Work out the finished part from the listing and answer in its coordinate system (mm). Round coordinates to 2 decimals unless told otherwise and drop trailing zeros. Answer as CSV lines item,"result". Start each with the question number.
Q1. Each of these flat-tipped pins is pushed along its axis until it touches: pin 1 Ø8 at (y, z) = (30, -14) entering from -X; pin 2 Ø1 at (x, y) = (-18, -7.5) entering from -Z; pin 3 Ø2 at (x, y) = (13.5, 8) entering from -Z. Where does it stop, or does it pass through?
Q2. The mould has two halves that part along Y. Classify faces 1 (the face through (10.77, 14.94, -18.58)), 2 (the face through (-20.194, 3.291, -18.385)), 3 (the face through (-5, 6, 0)), 4 (the face through (-36.205, 38.706, -26.871)): +Y half, -Y half, draft (parallel to the pull), parting line (faces both ways), or undercut.
Q3. Straight lines are drawn through the part: L1, parallel to X at y = 18.5, z = -50; L2, parallel to X at y = 30, z = -39; L3, parallel to Y at x = -18, z = -51. For each, find the intervals that lie inside material, in ascending order. Write a range as [from, to].
```python
from build123d import *

# Parameters (mm, degrees)
CYLINDER009_R               = 15
CYLINDER009_DEPTH           = 80
CYLINDER009_PLACEMENT_ANGLE = 39
BOX010_W                    = 44
BOX010_H                    = 8
BOX010_DEPTH                = 80
BOX010_PLACEMENT_ANGLE      = 42
CYLINDER010_R               = 1
CYLINDER010_DEPTH           = 10
CYLINDER010_PLACEMENT_ANGLE = 45
CYLINDER011_R               = 1
CYLINDER011_DEPTH           = 10
CYLINDER011_PLACEMENT_ANGLE = 45
BOX011_W                    = 20
BOX011_H                    = 11
BOX011_DEPTH                = 80
BOX011_PLACEMENT_ANGLE      = 45
CYLINDER007_R               = 8.5
CYLINDER007_DEPTH           = 45
BOX005_W                    = 100
BOX005_H                    = 200
BOX005_DEPTH                = 50
BOX005_PITCH_ANGLE          = 60
BOX005_PLACEMENT_ANGLE      = -45
BOX016_W                    = 100
BOX016_H                    = 100
BOX016_DEPTH                = 100
BOX016_PLACEMENT_ANGLE      = 45
BOX017_W                    = 100
BOX017_H                    = 100
BOX017_DEPTH                = 100
BOX017_PLACEMENT_ANGLE      = 45
BOX018_W                    = 200
BOX018_H                    = 200
BOX018_DEPTH                = 200
CONE003_ANGLE               = 180
CONE003_ROLL_ANGLE          = -90
CONE003_PLACEMENT_ANGLE     = -135
CONE002_ANGLE               = 180
CONE002_ROLL_ANGLE          = -90
CONE002_PLACEMENT_ANGLE     = -135
CYLINDER018_R               = 53
CYLINDER018_DEPTH           = 60
BOX019_W                    = 38
BOX019_H                    = 75
BOX019_DEPTH                = 63
BOX019_PLACEMENT_ANGLE      = 45
CYLINDER006_R               = 53
CYLINDER006_DEPTH           = 53
TUBE009_R                   = 8.5
TUBE009_R_2                 = 7
TUBE009_DEPTH               = 53


with BuildPart() as cylinder009:
    # Cylinder009 → Cylinder009 (new body)
    with BuildSketch(Plane.XY):
        Circle(CYLINDER009_R)
    extrude(amount=CYLINDER009_DEPTH)


with BuildPart() as cylinder009_1:
    # Cylinder009 placement: moved
    add(cylinder009.part.moved(Location((-5.423136, 5.902507, -91))).rotate(Axis((-5.423136, 5.902507, -91), (0, 0, 1)), CYLINDER009_PLACEMENT_ANGLE))


with BuildPart() as cube010:
    # Box010 → Box010 (new body)
    with BuildSketch(Plane.XY):
        with Locations((22, 4)):
            Rectangle(BOX010_W, BOX010_H)
    extrude(amount=BOX010_DEPTH)


with BuildPart() as cube010_1:
    # Box010 placement: moved
    add(cube010.part.moved(Location((-19.127921, -11.982839, -91))).rotate(Axis((-19.127921, -11.982839, -91), (0, 0, 1)), BOX010_PLACEMENT_ANGLE))


with BuildPart() as cone004:
    # Cone004 → Cone004 (revolve)
    with BuildSketch(Plane(origin=(0, 0, -53), x_dir=(1, 0, 0), z_dir=(0, -1, 0))):
        Polygon((0, 0), (51.5, 0), (20, 29), (0, 29), align=None)
    revolve(axis=Axis((0, 0, -53), (0, 0, 1)))


with BuildPart() as cylinder010:
    # Cylinder010 → Cylinder010 (new body)
    with BuildSketch(Plane.XY):
        Circle(CYLINDER010_R)
    extrude(amount=CYLINDER010_DEPTH)


with BuildPart() as cylinder010_1:
    # Cylinder010 placement: moved
    add(cylinder010.part.moved(Location((-18.384776, -7.071068, -11))).rotate(Axis((-18.384776, -7.071068, -11), (0, 0, 1)), CYLINDER010_PLACEMENT_ANGLE))


with BuildPart() as cylinder011:
    # Cylinder011 → Cylinder011 (new body)
    with BuildSketch(Plane.XY):
        Circle(CYLINDER011_R)
    extrude(amount=CYLINDER011_DEPTH)


with BuildPart() as cylinder011_1:
    # Cylinder011 placement: moved
    add(cylinder011.part.moved(Location((8.485281, 18.384776, -11))).rotate(Axis((8.485281, 18.384776, -11), (0, 0, 1)), CYLINDER011_PLACEMENT_ANGLE))


with BuildPart() as fusion010:
    # Box011 → Box011 (new body)
    with BuildSketch(Plane.XY):
        with Locations((10, 5.5)):
            Rectangle(BOX011_W, BOX011_H)
    extrude(amount=BOX011_DEPTH)


with BuildPart() as fusion010_1:
    # Box011 placement: moved
    add(fusion010.part.moved(Location((-19.79899, 7.071068, -91))).rotate(Axis((-19.79899, 7.071068, -91), (0, 0, 1)), BOX011_PLACEMENT_ANGLE))

    # Fusion010: union Cylinder009, Cube010, Cone004, Cylinder010, Cylinder011
    add(cylinder009_1.part)
    add(cube010_1.part)
    add(cone004.part)
    add(cylinder010_1.part)
    add(cylinder011_1.part)


with BuildPart() as cylinder007:
    # Cylinder007 → Cylinder007 (new body)
    with BuildSketch(Plane.XY.offset(-43)):
        Circle(CYLINDER007_R)
    extrude(amount=CYLINDER007_DEPTH)


with BuildPart() as cube005:
    # Box005 → Box005 (new body)
    with BuildSketch(Plane.XY):
        with Locations((50, 100)):
            Rectangle(BOX005_W, BOX005_H)
    extrude(amount=BOX005_DEPTH)


with BuildPart() as cube005_1:
    # Box005 pitch: moved
    add(cube005.part.rotate(Axis((0, 0, 0), (0, 1, 0)), BOX005_PITCH_ANGLE))


with BuildPart() as cube005_2:
    # Box005 placement: moved
    add(cube005_1.part.moved(Location((-38.183766, -91.923882, 0))).rotate(Axis((-38.183766, -91.923882, 0), (0, 0, 1)), BOX005_PLACEMENT_ANGLE))


with BuildPart() as cube016:
    # Box016 → Box016 (new body)
    with BuildSketch(Plane.XY):
        with Locations((50, 50)):
            Rectangle(BOX016_W, BOX016_H)
    extrude(amount=BOX016_DEPTH)


with BuildPart() as cube016_1:
    # Box016 placement: moved
    add(cube016.part.moved(Location((-71.320657, -123.15444, -92))).rotate(Axis((-71.320657, -123.15444, -92), (0, 0, -1)), BOX016_PLACEMENT_ANGLE))


with BuildPart() as cube017:
    # Box017 → Box017 (new body)
    with BuildSketch(Plane.XY):
        with Locations((50, 50)):
            Rectangle(BOX017_W, BOX017_H)
    extrude(amount=BOX017_DEPTH)


with BuildPart() as cube017_1:
    # Box017 placement: moved
    add(cube017.part.moved(Location((53.030932, 0.040624, -92))).rotate(Axis((53.030932, 0.040624, -92), (0, 0, -1)), BOX017_PLACEMENT_ANGLE))


with BuildPart() as cube018:
    # Box018 → Box018 (new body)
    with BuildSketch(Plane(origin=(-111, -128, -263), x_dir=(1, 0, 0), z_dir=(0, 0, 1))):
        with Locations((100, 100)):
            Rectangle(BOX018_W, BOX018_H)
    extrude(amount=BOX018_DEPTH)


with BuildPart() as fusion009004:
    # Cone003 → Cone003 (revolve)
    with BuildSketch(Plane.XZ):
        Polygon((0, 0), (2, 0), (78, 80), (0, 80), align=None)
    revolve(axis=Axis((0, 0, 0), (0, 0, 1)), revolution_arc=CONE003_ANGLE)


with BuildPart() as fusion009004_1:
    # Cone003 roll: moved
    add(fusion009004.part.rotate(Axis((0, 0, 0), (1, 0, 0)), CONE003_ROLL_ANGLE))


with BuildPart() as fusion009004_2:
    # Cone003 placement: moved
    add(fusion009004_1.part.rotate(Axis((0, 0, 0), (0, 0, 1)), CONE003_PLACEMENT_ANGLE))

    # Fusion009004: union Cube016, Cube017, Cube018
    add(cube016_1.part)
    add(cube017_1.part)
    add(cube018.part)


with BuildPart() as obj1:
    # Cone002 → Cone002 (revolve)
    with BuildSketch(Plane.XZ):
        Polygon((0, 0), (2, 0), (80, 80), (0, 80), align=None)
    revolve(axis=Axis((0, 0, 0), (0, 0, 1)), revolution_arc=CONE002_ANGLE)


with BuildPart() as obj1_1:
    # Cone002 roll: moved
    add(obj1.part.rotate(Axis((0, 0, 0), (1, 0, 0)), CONE002_ROLL_ANGLE))


with BuildPart() as obj1_2:
    # Cone002 placement: moved
    add(obj1_1.part.rotate(Axis((0, 0, 0), (0, 0, 1)), CONE002_PLACEMENT_ANGLE))


with BuildPart() as cut007:
    # Cut004 base: copy of obj1
    add(obj1_2.part)

    # Cut004: cut Fusion009004
    add(fusion009004_2.part, mode=Mode.SUBTRACT)

    # Cut007: cut Cube005
    add(cube005_2.part, mode=Mode.SUBTRACT)


with BuildPart() as cylinder018:
    # Cylinder018 → Cylinder018 (new body)
    with BuildSketch(Plane.XY.offset(-63)):
        Circle(CYLINDER018_R)
    extrude(amount=CYLINDER018_DEPTH)


with BuildPart() as cut009005:
    # Box019 → Box019 (new body)
    with BuildSketch(Plane.XY):
        with Locations((19, 37.5)):
            Rectangle(BOX019_W, BOX019_H)
    extrude(amount=BOX019_DEPTH)


with BuildPart() as cut009005_1:
    # Box019 placement: moved
    add(cut009005.part.moved(Location((-0.609979, -52.443762, -63))).rotate(Axis((-0.609979, -52.443762, -63), (0, 0, -1)), BOX019_PLACEMENT_ANGLE))

    # Cut009005: cut Cylinder018
    add(cylinder018.part, mode=Mode.SUBTRACT)


with BuildPart() as cut006:
    # Cylinder006 → Cylinder006 (new body)
    with BuildSketch(Plane.XY.offset(-53)):
        Circle(CYLINDER006_R)
    extrude(amount=CYLINDER006_DEPTH)

    # Fusion009005: union Cut009005
    add(cut009005_1.part)

    # Cut005: cut obj1
    add(obj1_2.part, mode=Mode.SUBTRACT)

    # Fusion005: union Cut007
    add(cut007.part)

    # Cut006: cut Cylinder007
    add(cylinder007.part, mode=Mode.SUBTRACT)


with BuildPart() as cut009_middle:
    # Tube009 → Tube009 (new body)
    with BuildSketch(Plane.XY.offset(-53)):
        Circle(TUBE009_R)
        Circle(TUBE009_R_2, mode=Mode.SUBTRACT)
    extrude(amount=TUBE009_DEPTH)

    # Fusion006: union Cut006
    add(cut006.part)

    # Cut009: cut Fusion010
    add(fusion010_1.part, mode=Mode.SUBTRACT)


solid = cut009_middle.part
```
Findings:
1,pin 1,"stops at x = -46.18"
1,pin 2,"stops at z = -11"
1,pin 3,"stops at z = -24"
2,face 1,"undercut"
2,face 2,"undercut"
2,face 3,"draft"
2,face 4,"parting line"
3,L1,"x = [-49.67, -44.55], [44.55, 49.67]"
3,L2,"x = [-43.69, -20.43], [20.43, 43.69]"
3,L3,"y = [-49.85, -45.93], [45.93, 49.85]"
